from build123d import *

# Parameters (mm, degrees)
ESQUISSE1_W                                 = 100
ESQUISSE1_H                                 = 110
BOSS_EXTRU_1_DEPTH                          = 2
ESQUISSE3_W                                 = 100
ESQUISSE3_H                                 = 20
BOSS_EXTRU_2_DEPTH                          = 3
ESQUISSE6_R                                 = 2
ENL_V_MAT_EXTRU_1_DEPTH                     = 78.517739905
ENL_V_MAT_EXTRU_2_DEPTH                     = 78.517739905
CONG_2_R                                    = 10
BOSS_EXTRU_3_DEPTH                          = 3
FRAISAGE_POUR_VIS_T_TE_FRAIS_E_M51_AT_COUNT = 2
FRAISAGE_POUR_VIS_T_TE_FRAIS_E_M51_AT_PITCH = 80
BOSS_EXTRU_4_DEPTH                          = 65
BOSS_EXTRU_5_DEPTH                          = 2
CONG_3_R                                    = 7
D_GAGEMENT_M21_D                            = 2.4
D_GAGEMENT_M21_ON_FACE_2_D                  = 2.4
CONG_1_R                                    = 2


with BuildPart() as part:
    # Esquisse1 → Boss.-Extru.1 (new body)
    with BuildSketch(Plane.XY):
        Rectangle(ESQUISSE1_W, ESQUISSE1_H)
    extrude(amount=BOSS_EXTRU_1_DEPTH)

    # Esquisse3 → Boss.-Extru.2 (add)
    with BuildSketch(Plane.XZ.offset(55)):
        with Locations((0, -10)):
            Rectangle(ESQUISSE3_W, ESQUISSE3_H)
    extrude(amount=-BOSS_EXTRU_2_DEPTH)

    # Esquisse6 → Enlèv. mat.-Extru.1 (cut, through all)
    with BuildSketch(Plane.XY.offset(2)):
        with Locations((-43.5, 48.5)):
            Circle(ESQUISSE6_R)
        with Locations((43.5, 48.5)):
            Circle(ESQUISSE6_R)
        with Locations((-43.5, -38.5)):
            Circle(ESQUISSE6_R)
        with Locations((43.5, -38.5)):
            Circle(ESQUISSE6_R)
    extrude(amount=-ENL_V_MAT_EXTRU_1_DEPTH, mode=Mode.SUBTRACT)

    # Esquisse7 → Enlèv. mat.-Extru.2 (cut, through all)
    with BuildSketch(Plane.XY.offset(2)):
        with BuildLine():
            Line((0, 55), (-43.500000007, 55))
            ThreePointArc((-43.500000007, 55), (-41.012557693, 54.505216963), (-38.903805922, 53.096194078))
            Line((-38.903805922, 53.096194078), (0, 14.192388155))
            Line((0, 14.192388155), (0, 55))
        make_face()
        with BuildLine():
            Line((-9.192388155, 5), (-48.096194078, 43.903805922))
            ThreePointArc((-48.096194078, 43.903805922), (-49.505216961, 46.01255769), (-50, 48.5))
            Line((-50, 48.5), (-50, -38.5))
            ThreePointArc((-50, -38.5), (-49.505216961, -36.01255769), (-48.096194078, -33.903805922))
            Line((-48.096194078, -33.903805922), (-9.192388155, 5))
        make_face()
        with BuildLine():
            Line((-50, 55), (-50, 48.5))
            ThreePointArc((-50, 48.5), (-48.09619408, 53.096194075), (-43.500000007, 55))
            Line((-43.500000007, 55), (-50, 55))
        make_face()
    enl_v_mat_extru_2 = extrude(amount=-ENL_V_MAT_EXTRU_2_DEPTH, mode=Mode.SUBTRACT)

    # Symétrie1: Enlèv. mat.-Extru.2 across plane
    add(enl_v_mat_extru_2.mirror(Plane(origin=(0, 0, 0), x_dir=(0, 0, 1), z_dir=(1, 0, 0))), mode=Mode.SUBTRACT)

    # Congé2
    cong_2_edges = [part.edges().sort_by_distance(p)[0] for p in [
        (9.192388155, 5, 1),
        (-9.192388155, 5, 1),
        (0, 14.192388155, 1),
    ]]
    fillet(cong_2_edges, radius=CONG_2_R)

    # Esquisse8 → Boss.-Extru.3 (add)
    with BuildSketch(Plane.XZ.offset(55)):
        Polygon((50, 2), (69.091883092, -17.091883092), (66.183766184, -20), (50, -20), align=None)
    extrude(amount=-BOSS_EXTRU_3_DEPTH)

    # Esquisse5 → Fraisage pour vis à tête fraisée M51 (revolve, cut)
    with BuildSketch(Plane(origin=(-33, -52, -12), x_dir=(0, 0, 1), z_dir=(1, 0, 0))):
        Polygon((0, 0), (0, 3), (2.75, 3), (2.75, 2.45), (5.2, 0), align=None)
    fraisage_pour_vis_t_te_frais_e_m51 = revolve(axis=Axis((-33, -45.65, -12), (0, -1, 0)), mode=Mode.SUBTRACT)

    # Fraisage pour vis à tête fraisée M51 at: Fraisage pour vis à tête fraisée M51 ×2
    with Locations(*[(i * FRAISAGE_POUR_VIS_T_TE_FRAIS_E_M51_AT_PITCH, 0, 0) for i in range(1, FRAISAGE_POUR_VIS_T_TE_FRAIS_E_M51_AT_COUNT)]):
        add(fraisage_pour_vis_t_te_frais_e_m51, mode=Mode.SUBTRACT)

    # Esquisse9 → Boss.-Extru.4 (add)
    with BuildSketch(Plane(origin=(0, -52, 0), x_dir=(1, 0, 0), z_dir=(0, 1, 0))):
        Polygon((50, -2), (69.091883092, 17.091883092), (68.091883092, 18.091883092), (50, 0), align=None)
    extrude(amount=BOSS_EXTRU_4_DEPTH)

    # Esquisse10 → Boss.-Extru.5 (add)
    with BuildSketch(Plane.XY.offset(2)):
        Polygon((48.096194078, -33.903805922), (50, -35.807611845), (50, -38.5), align=None)
    extrude(amount=-BOSS_EXTRU_5_DEPTH)

    # Congé3
    # the kernel refuses this fillet: 7 mm, written as the material it adds along each edge
    with BuildSketch(Plane(origin=(50, -35.807611845, 2), x_dir=(-0.707106781186548, 0.7071067811865469, 0), z_dir=(0, 0, -1))) as cong_3_piece_1_section:
        with BuildLine():
            CenterArc((CONG_3_R * 2.41421356237, CONG_3_R), CONG_3_R, 135, 135)
            Line((CONG_3_R * 1.70710678119, CONG_3_R * 1.70710678119), (0, 0))
            Line((0, 0), (CONG_3_R * 2.41421356237, 0))
        make_face()
    cong_3_piece_1 = extrude(amount=2, mode=Mode.PRIVATE)
    cong_3_piece_1 = split(cong_3_piece_1, bisect_by=Plane(origin=(49.112602223, -28.296939532, 0.887397777), z_dir=(0.7071067811865487, 0, 0.7071067811865464)), keep=Keep.TOP, mode=Mode.PRIVATE)
    cong_3_piece_1 = split(cong_3_piece_1, bisect_by=Plane(origin=(50.112602223, -28.296939532, 1.887397777), z_dir=(-0.7071067811865483, 0, -0.7071067811865467)), keep=Keep.TOP, mode=Mode.PRIVATE)
    add(cong_3_piece_1)
    with BuildSketch(Plane(origin=(50, -35.807611845, 2), x_dir=(-0.707106781186548, 0.7071067811865469, 0), z_dir=(0, 0, -1))) as cong_3_piece_2_section:
        with BuildLine():
            CenterArc((CONG_3_R * 2.41421356237, CONG_3_R), CONG_3_R, 135, 135)
            Line((CONG_3_R * 1.70710678119, CONG_3_R * 1.70710678119), (0, 0))
            Line((0, 0), (CONG_3_R * 2.41421356237, 0))
        make_face()
    cong_3_piece_2 = extrude(amount=2, mode=Mode.PRIVATE)
    cong_3_piece_2 = split(cong_3_piece_2, bisect_by=Plane(origin=(47.570771883, -28.332960354, 2.429228117), z_dir=(-0.7071067811865487, 0, -0.7071067811865464)), keep=Keep.TOP, mode=Mode.PRIVATE)
    add(cong_3_piece_2)

    # Dégagement M21 (through all)
    with Locations(Plane(origin=(52.828427125, 7, -0.828427125), x_dir=(-0.707106781187, 0, 0.707106781187), z_dir=(0.707106781187, 0, 0.707106781187))):
        with Locations((0, 0)):
            Hole(D_GAGEMENT_M21_D / 2)

    # Dégagement M21 on face 2 (through all)
    with Locations(Plane(origin=(66.263455967, 7, -14.263455967), x_dir=(0.707106781187, 0, -0.707106781187), z_dir=(0.707106781187, 0, 0.707106781187))):
        with Locations((0, 0), (0, -56), (-19, -56)):
            Hole(D_GAGEMENT_M21_ON_FACE_2_D / 2)

    # Congé1
    cong_1_edges = [part.edges().sort_by_distance(p)[0] for p in [
        (0, -52, 0),
        (59.045941546, -52, -9.045941546),
    ]]
    fillet(cong_1_edges, radius=CONG_1_R)


solid = part.part
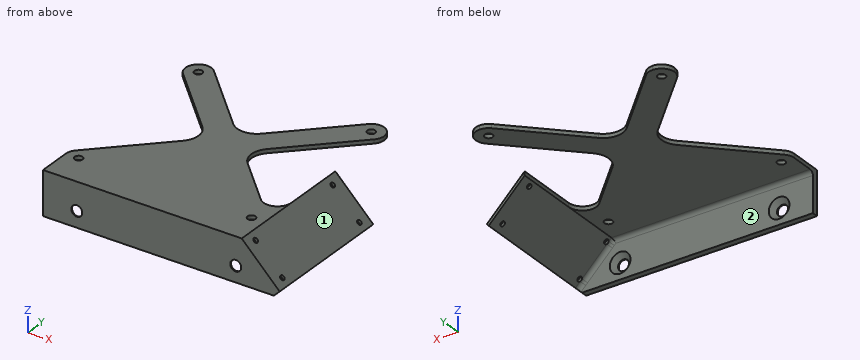
Part model, mm, in its own coordinate system. Face numbers are marked on the shaded views. A direction names the side the tool comes from. Give positions to 0.01 mm unless a question says otherwise; leave off trailing zeros. Order: outer loops, then holes, each group sorted by start corner. A loop starts at its lowest first (then second) coordinate and runs counter-clockwise, first axis right, second up. Notation, with made-up numbers: (-8.75, 10) - (-2.75, 10) arc R19 cw to (-2.75, 17) - close; hole circle Ø11 at (-20, 16.5). An arc over 180 degrees is marked (long way). Use a Markdown table: item, result.
1) Saw through at B-B on y = 0.5. List the corners of the cut face in (x, z).
Checked values:
| item | result |
|---|---|
| outline | (-14.4, 0) - (14.4, 0) - (14.4, 2) - (-14.4, 2) - close; (50, 0) - (68.09, -18.09) - (69.09, -17.09) - (50, 2) - close |
2) Saw through at D-D on z = -12. Count the separate pieces of the cut face and the enclosed holes in it, plus the area to 3 significant figures.
Checked values:
| item | result |
|---|---|
| separate pieces | 3 |
| enclosed holes | 0 |
| area | 428 mm² |
3) Flat gauge pins, fed straight in: P1, Ø6.5, axis at x = -43.5, y = 48.5, coming from the -Z side; P2, Ø9, axis at x = 24.5, z = -10.5, coming from the +Y side; P3, Ø8, axis at x = -2.5, y = 24.5, coming from the +Z side; P4, Ø1, axis at y = 11, z = -1, coming from the -X side. Where does each tip first touch, or does it go through?
Checked values:
| item | result |
|---|---|
| P1 | z = 0 |
| P2 | y = -52 |
| P3 | through |
| P4 | x = 50.5 |
4) 3-axis set-ups, long thin cutter, end or side, ignore diameter. For the marked faces 1 and 2: which of +Z, -Z, +X, -X, +Y, -Y reach the whole face in a straight line?
Checked values:
| item | result |
|---|---|
| face 1 | +Z, +X, +Y, -Y |
| face 2 | -Z, -X, +Y |
5) Probe L1, parallel to Z at x = 33, y = 40.5; L2, parallel to Y at x = 33.5, z = -3.75; L3, parallel to Y at x = -43.5, z = 0.9. List the from-to ranges inside material, lowest first. Write a range as from..to.
Checked values:
| item | result |
|---|---|
| L1 | 0..2 |
| L2 | -55..-52 |
| L3 | -55..-40.5, -36.5..-29.31, 39.31..46.5, 50.5..55 |
6) Saw through at C-C on x = -2. List the corners of the cut face in (y, z).
Checked values:
| item | result |
|---|---|
| outline | (-55, -20) - (-52, -20) - (-52, -2) arc R2 cw to (-50, 0) - (18.54, 0) - (18.54, 2) - (-55, 2) - close |
7) Saw through at A-A on x = -33. List the corners of the cut face in (y, z), plus the area to 3 significant figures.
Checked values:
| item | result |
|---|---|
| outline | (-55, -20) - (-52, -20) - (-52, -17.2) - (-54.45, -14.75) - (-55, -14.75) - close; (-55, -9.25) - (-54.45, -9.25) - (-52, -6.8) - (-52, -2) arc R2 cw to (-50, 0) - (-18.81, 0) - (-18.81, 2) - (-55, 2) - close; (28.81, 0) - (47.19, 0) - (47.19, 2) - (28.81, 2) - close |
| area | 148 mm² |
